Design review of the part built by this model. Coordinates are the model's own, in mm. Coordinates: 2 decimals unless noted, no trailing zeros. Loops run counter-clockwise (first coordinate to the right, second up) from the corner with the lowest first, then second, coordinate; pieces in that order, holes last. Notation, with made-up numbers: (59.5, 78) -> (71.5, 78) arc R28 ccw to (71.5, 101) -> close; hole circle Ø9 at (41.5, 72). An arc over 180 degrees is marked (long way). Use a Markdown table: item, result. Add a question column.
Q1. For probe 1 along X at (y, z) = (-2.5, 0.25); probe 2 along X at (y, z) = (-1, 0.4); probe 3 along Y at (x, z) = (60, 0.3), list the stretches that pass through material, from the lowest coordinate up.
Q2. Take a section at B-B on z = 0.4. Write out the cut boundary in (x, y).
Q3. Take a section at A-A on y = 0. Write out the cut boundary in (x, z).
Q4. Take a section at C-C on x = 95. Write out the cut boundary in (y, z), plus the area to 3 significant figures.
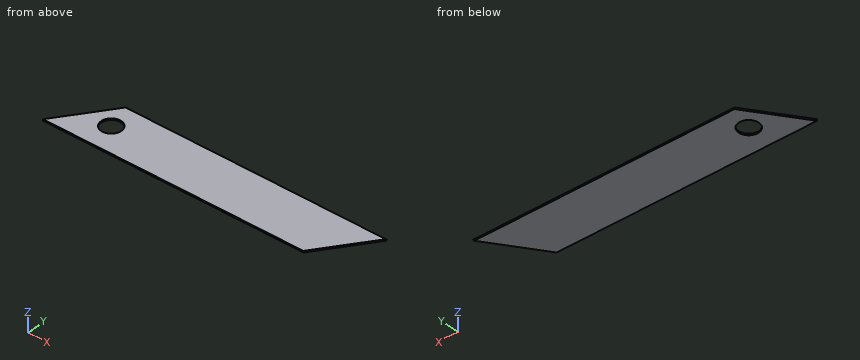
from build123d import *

# Parameters (mm, degrees)
F0_R        = 3.341537713
F1_DEPTH    = 0.5
F2_T1_DEPTH = 89.571682988


# Not quite as in the source:
# - a fillet or chamfer that OpenCascade refuses, or shapes differently, is made with other operations: its cross-section is extruded or revolved along the edge and cut away or added


with BuildPart() as f1:
    # F0 (on Top) → F1 (new body)
    with BuildSketch(Plane.XY):
        Polygon((16.2269707607, 8.9300729632), (3.6232350729, -9.0699270368), (90.6232350729, -9.0699270368), (103.2269707607, 8.9300729632), align=None)
        with Locations((18.4976458549, 0)):
            Circle(F0_R, mode=Mode.SUBTRACT)
    extrude(amount=F1_DEPTH)

    # F2: chamfer of 0.5 on 2 edges, made by hand

    # F2_s2 → F2_t1 (cut)
    with BuildSketch(Plane.YZ.offset(14.9411292667)):
        Polygon((8.9300729632, 0), (8.4300729632, 0.5), (8.9300729632, 0.5), align=None)
        Polygon((8.9300729632, 0.5), (8.4300729632, 0), (8.9300729632, 0), align=None)
    extrude(amount=F2_T1_DEPTH, mode=Mode.SUBTRACT)


solid = f1.part
Answer list:
| question | item | result |
|---|---|---|
| 1 | probe 1 | 8.22 to 16.28, 20.71 to 95.22 |
| 1 | probe 2 | 9.27 to 15.31, 21.69 to 96.27 |
| 1 | probe 3 | -9.07 to 8.63 |
| 2 | outline | (3.62, -9.07) -> (90.62, -9.07) -> (102.95, 8.53) -> (15.95, 8.53) -> close; hole circle Ø6.68 at (18.5, 0) |
| 3 | outline | (9.97, 0) -> (15.16, 0) -> (15.16, 0.5) -> (9.97, 0.5) -> close; (21.84, 0) -> (96.97, 0) -> (96.97, 0.5) -> (21.84, 0.5) -> close |
| 4 | outline | (-2.82, 0) -> (8.43, 0) -> (8.68, 0.25) -> (8.43, 0.5) -> (-2.82, 0.5) -> close |
| 4 | area | 5.69 mm² |
